from build123d import *

# Parameters (mm, degrees)
SKIZZE1_W                       = 21.482125196
SKIZZE1_H                       = 3.731950896
AUFSATZ_LINEAR_AUSTRAGEN1_DEPTH = 0.2
SKIZZE2_W                       = 21.482125196
SKIZZE2_H                       = 0.1
SCHNITT_LINEAR_AUSTRAGEN1_DEPTH = 0.1
SKIZZE3_R                       = 0.4
SCHNITT_LINEAR_AUSTRAGEN2_DEPTH = 1.2
LINEARES_MUSTER1_COUNT          = 4
LINEARES_MUSTER1_PITCH          = 5


with BuildPart() as part:
    # Skizze1 → Aufsatz-Linear austragen1 (new body)
    with BuildSketch(Plane.XY):
        Rectangle(SKIZZE1_W, SKIZZE1_H)
    extrude(amount=AUFSATZ_LINEAR_AUSTRAGEN1_DEPTH)

    # Skizze2 → Schnitt-Linear austragen1 (cut)
    with BuildSketch(Plane.XY.offset(0.2)):
        Rectangle(SKIZZE2_W, SKIZZE2_H)
    extrude(amount=-SCHNITT_LINEAR_AUSTRAGEN1_DEPTH, mode=Mode.SUBTRACT)

    # Skizze3 → Schnitt-Linear austragen2 (cut, through all)
    with BuildSketch(Plane.XY.offset(0.2)):
        with Locations((9.957181888, -0.562943668)):
            Circle(SKIZZE3_R)
        with Locations((8.850641756, -1.365185264)):
            Circle(SKIZZE3_R)
        with Locations((9.957181888, 0.571259967)):
            Circle(SKIZZE3_R)
        with Locations((8.850641756, 1.359669812)):
            Circle(SKIZZE3_R)
    schnitt_linear_austragen2 = extrude(amount=-SCHNITT_LINEAR_AUSTRAGEN2_DEPTH, mode=Mode.SUBTRACT)

    # Lineares Muster1: Schnitt-Linear austragen2 ×4
    with Locations(*[(-i * LINEARES_MUSTER1_PITCH, 0, 0) for i in range(1, LINEARES_MUSTER1_COUNT)]):
        add(schnitt_linear_austragen2, mode=Mode.SUBTRACT)


solid = part.part
Geometry: final body of the model. Coordinates: model frame, mm. Give positions to 0.01 mm unless a question says otherwise; leave off trailing zeros. Write each loop counter-clockwise with the first axis right and the second up, starting at its lowest first coordinate (ties: lowest second). Pieces come first, ordered by that corner, then holes. Notation, with made-up numbers: (-11.75, -2) -> (45.25, -2) arc R25 ccw to (45.25, 21) -> close; hole circle Ø4 at (26.25, 23.25). An arc over 180 degrees is marked (long way). Answer in a Markdown table with one row per item.
(1) Section query A-A on z = 0.15. State how many separate pieces and enclosed holes the cut face has, then the cut area to 3 significant figures.
Answers below:
| item | result |
|---|---|
| separate pieces | 2 |
| enclosed holes | 16 |
| area | 70.0 mm^2 |
(2) Section query B-B on x = 0. Return loops of the section in (y, z), then the cut area to 3 significant figures.
Answers below:
| item | result |
|---|---|
| outline | (-1.87, 0) -> (-0.96, 0) -> (-0.96, 0.2) -> (-1.87, 0.2) -> close; (-0.17, 0) -> (0.17, 0) -> (0.17, 0.2) -> (0.05, 0.2) -> (0.05, 0.1) -> (-0.05, 0.1) -> (-0.05, 0.2) -> (-0.17, 0.2) -> close; (0.97, 0) -> (1.87, 0) -> (1.87, 0.2) -> (0.97, 0.2) -> close |
| area | 0.418 mm^2 |
(3) Ray query, line 1 along X through (y, z) = (-1.4, 0.05); line 2 along X through (y, z) = (-1.1, 0.1). Return the intervals inside material, ascending. Write a range as [from, to].
Answers below:
| item | result |
|---|---|
| line 1 | [-10.74, -6.55], [-5.75, -1.55], [-0.75, 3.45], [4.25, 8.45], [9.25, 10.74] |
| line 2 | [-10.74, -6.45], [-5.85, -1.45], [-0.85, 3.55], [4.15, 8.55], [9.15, 10.74] |
